Could you check a few things on this model? Use its own coordinates, in mm. Face numbers are marked on the shaded views. A direction names the side the tool comes from. Give positions to 0.01 mm unless a question says otherwise; leave off trailing zeros. Loops run counter-clockwise (first coordinate to the right, second up) from the corner with the lowest first, then second, coordinate; pieces in that order, holes last. Notation, with made-up numbers: M 17.5,-2.5 L 66.5,-2.5 A25 ccw 66.5,12.5 Z; hole C 27.25,24.5 d5. An arc over 180 degrees is marked long. Use CSV: the item, a comma, the result in double quotes.
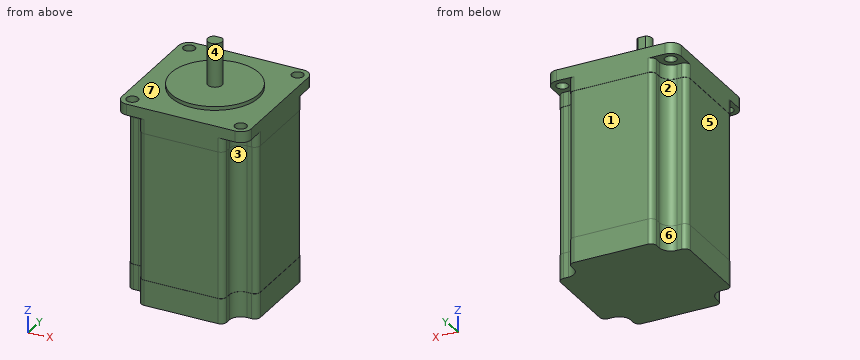
```python
from build123d import *

# Parameters (mm, degrees)
SKETCH1_R           = 3.175
BOSS_EXTRUDE1_DEPTH = 20.6
SKETCH2_R           = 19.05
BOSS_EXTRUDE2_DEPTH = 1.6
BOSS_EXTRUDE3_DEPTH = 4.8
BOSS_EXTRUDE4_DEPTH = 81.2
SKETCH7_W           = 3.420526276
SKETCH7_H           = 1.112659396
CUT_EXTRUDE5_DEPTH  = 15
CUT_EXTRUDE6_REACH  = 88
SKETCH8_R           = 2.55
CUT_EXTRUDE7_DEPTH  = 32


with BuildPart() as part:
    # Sketch1 → Boss-Extrude1 (new body)
    with BuildSketch(Plane.XY):
        Circle(SKETCH1_R)
    extrude(amount=BOSS_EXTRUDE1_DEPTH)

    # Sketch2 → Boss-Extrude2 (add)
    with BuildSketch(Plane(origin=(0, 0, 0), x_dir=(-1, 0, 0), z_dir=(0, 0, -1))):
        Circle(SKETCH2_R)
    extrude(amount=-BOSS_EXTRUDE2_DEPTH)

    # Sketch3 → Boss-Extrude3 (add)
    with BuildSketch(Plane(origin=(0, 0, 0), x_dir=(-1, 0, 0), z_dir=(0, 0, -1))):
        with BuildLine():
            Line((23.6, -28.2), (-23.6, -28.2))
            ThreePointArc((-23.6, -28.2), (-26.852691193, -26.852691193), (-28.2, -23.6))
            Line((-28.2, -23.6), (-28.2, 23.6))
            ThreePointArc((-28.2, 23.6), (-26.852691193, 26.852691193), (-23.6, 28.2))
            Line((-23.6, 28.2), (23.6, 28.2))
            ThreePointArc((23.6, 28.2), (26.852691193, 26.852691193), (28.2, 23.6))
            Line((28.2, 23.6), (28.2, -23.6))
            ThreePointArc((28.2, -23.6), (26.852691193, -26.852691193), (23.6, -28.2))
        make_face()
    extrude(amount=BOSS_EXTRUDE3_DEPTH)

    # Sketch4 → Boss-Extrude4 (add)
    with BuildSketch(Plane(origin=(0, 0, -4.8), x_dir=(-1, 0, 0), z_dir=(0, 0, -1))):
        with BuildLine():
            Line((-18.57, 23.57), (-18.57, 25.7))
            ThreePointArc((-18.57, 25.7), (-17.837766953, 27.467766953), (-16.07, 28.2))
            Line((-16.07, 28.2), (16.07, 28.2))
            ThreePointArc((16.07, 28.2), (17.837766953, 27.467766953), (18.57, 25.7))
            Line((18.57, 25.7), (18.57, 23.57))
            ThreePointArc((18.57, 23.57), (20.034466094, 20.034466094), (23.57, 18.57))
            Line((23.57, 18.57), (25.7, 18.57))
            ThreePointArc((25.7, 18.57), (27.467766953, 17.837766953), (28.2, 16.07))
            Line((28.2, 16.07), (28.2, -16.07))
            ThreePointArc((28.2, -16.07), (27.467766953, -17.837766953), (25.7, -18.57))
            Line((25.7, -18.57), (23.57, -18.57))
            ThreePointArc((23.57, -18.57), (20.034466094, -20.034466094), (18.57, -23.57))
            Line((18.57, -23.57), (18.57, -25.7))
            ThreePointArc((18.57, -25.7), (17.837766953, -27.467766953), (16.07, -28.2))
            Line((16.07, -28.2), (-16.07, -28.2))
            ThreePointArc((-16.07, -28.2), (-17.837766953, -27.467766953), (-18.57, -25.7))
            Line((-18.57, -25.7), (-18.57, -23.57))
            ThreePointArc((-18.57, -23.57), (-20.034466094, -20.034466094), (-23.57, -18.57))
            Line((-23.57, -18.57), (-25.7, -18.57))
            ThreePointArc((-25.7, -18.57), (-27.467766953, -17.837766953), (-28.2, -16.07))
            Line((-28.2, -16.07), (-28.2, 16.07))
            ThreePointArc((-28.2, 16.07), (-27.467766953, 17.837766953), (-25.7, 18.57))
            Line((-25.7, 18.57), (-23.57, 18.57))
            ThreePointArc((-23.57, 18.57), (-20.034466094, 20.034466094), (-18.57, 23.57))
        make_face()
    extrude(amount=BOSS_EXTRUDE4_DEPTH)

    # Sketch7 → Cut-Extrude5 (cut)
    with BuildSketch(Plane.XY.offset(20.6)):
        with Locations((0, 3.231329698)):
            Rectangle(SKETCH7_W, SKETCH7_H)
    extrude(amount=-CUT_EXTRUDE5_DEPTH, mode=Mode.SUBTRACT)

    # Sketch8 → Cut-Extrude6 (cut, up to next)
    with BuildSketch(Plane.XY, mode=Mode.PRIVATE) as cut_extrude6_sk1:
        with Locations((-23.57, 23.57)):
            Circle(SKETCH8_R)
    cut_extrude6_tool1 = extrude(cut_extrude6_sk1.sketch, amount=-CUT_EXTRUDE6_REACH, mode=Mode.PRIVATE) & part.part
    add(cut_extrude6_tool1.solids().sort_by_distance((-23.57, 23.57, 0))[0], mode=Mode.SUBTRACT)
    # Sketch8 → Cut-Extrude6 (cut, up to next)
    with BuildSketch(Plane.XY, mode=Mode.PRIVATE) as cut_extrude6_sk2:
        with Locations((23.57, 23.57)):
            Circle(SKETCH8_R)
    cut_extrude6_tool2 = extrude(cut_extrude6_sk2.sketch, amount=-CUT_EXTRUDE6_REACH, mode=Mode.PRIVATE) & part.part
    add(cut_extrude6_tool2.solids().sort_by_distance((23.57, 23.57, 0))[0], mode=Mode.SUBTRACT)
    # Sketch8 → Cut-Extrude6 (cut, up to next)
    with BuildSketch(Plane.XY, mode=Mode.PRIVATE) as cut_extrude6_sk3:
        with Locations((23.57, -23.57)):
            Circle(SKETCH8_R)
    cut_extrude6_tool3 = extrude(cut_extrude6_sk3.sketch, amount=-CUT_EXTRUDE6_REACH, mode=Mode.PRIVATE) & part.part
    add(cut_extrude6_tool3.solids().sort_by_distance((23.57, -23.57, 0))[0], mode=Mode.SUBTRACT)
    # Sketch8 → Cut-Extrude6 (cut, up to next)
    with BuildSketch(Plane.XY, mode=Mode.PRIVATE) as cut_extrude6_sk4:
        with Locations((-23.57, -23.57)):
            Circle(SKETCH8_R)
    cut_extrude6_tool4 = extrude(cut_extrude6_sk4.sketch, amount=-CUT_EXTRUDE6_REACH, mode=Mode.PRIVATE) & part.part
    add(cut_extrude6_tool4.solids().sort_by_distance((-23.57, -23.57, 0))[0], mode=Mode.SUBTRACT)

    # Sketch9 → Cut-Extrude7 (cut, symmetric)
    with BuildSketch(Plane.XY.offset(-43)):
        with BuildLine():
            Line((18.57, 23.57), (18.57, 25.7))
            ThreePointArc((18.57, 25.7), (17.837766953, 27.467766953), (16.07, 28.2))
            Line((16.07, 28.2), (-16.07, 28.2))
            ThreePointArc((-16.07, 28.2), (-17.837766953, 27.467766953), (-18.57, 25.7))
            Line((-18.57, 25.7), (-18.57, 23.57))
            ThreePointArc((-18.57, 23.57), (-20.034466094, 20.034466094), (-23.57, 18.57))
            Line((-23.57, 18.57), (-25.7, 18.57))
            ThreePointArc((-25.7, 18.57), (-27.467766953, 17.837766953), (-28.2, 16.07))
            Line((-28.2, 16.07), (-28.2, -16.07))
            ThreePointArc((-28.2, -16.07), (-27.467766953, -17.837766953), (-25.7, -18.57))
            Line((-25.7, -18.57), (-23.57, -18.57))
            ThreePointArc((-23.57, -18.57), (-20.034466094, -20.034466094), (-18.57, -23.57))
            Line((-18.57, -23.57), (-18.57, -25.7))
            ThreePointArc((-18.57, -25.7), (-17.837766953, -27.467766953), (-16.07, -28.2))
            Line((-16.07, -28.2), (16.07, -28.2))
            ThreePointArc((16.07, -28.2), (17.837766953, -27.467766953), (18.57, -25.7))
            Line((18.57, -25.7), (18.57, -23.57))
            ThreePointArc((18.57, -23.57), (20.034466094, -20.034466094), (23.57, -18.57))
            Line((23.57, -18.57), (25.7, -18.57))
            ThreePointArc((25.7, -18.57), (27.467766953, -17.837766953), (28.2, -16.07))
            Line((28.2, -16.07), (28.2, 16.07))
            ThreePointArc((28.2, 16.07), (27.467766953, 17.837766953), (25.7, 18.57))
            Line((25.7, 18.57), (23.57, 18.57))
            ThreePointArc((23.57, 18.57), (20.034466094, 20.034466094), (18.57, 23.57))
        make_face()
        with BuildLine():
            Line((18.47, 23.57), (18.47, 25.7))
            ThreePointArc((18.47, 25.7), (17.767056275, 27.397056275), (16.07, 28.1))
            Line((16.07, 28.1), (-16.07, 28.1))
            ThreePointArc((-16.07, 28.1), (-17.767056275, 27.397056275), (-18.47, 25.7))
            Line((-18.47, 25.7), (-18.47, 23.57))
            ThreePointArc((-18.47, 23.57), (-19.963755416, 19.963755416), (-23.57, 18.47))
            Line((-23.57, 18.47), (-25.7, 18.47))
            ThreePointArc((-25.7, 18.47), (-27.397056275, 17.767056275), (-28.1, 16.07))
            Line((-28.1, 16.07), (-28.1, -16.07))
            ThreePointArc((-28.1, -16.07), (-27.397056275, -17.767056275), (-25.7, -18.47))
            Line((-25.7, -18.47), (-23.57, -18.47))
            ThreePointArc((-23.57, -18.47), (-19.963755416, -19.963755416), (-18.47, -23.57))
            Line((-18.47, -23.57), (-18.47, -25.7))
            ThreePointArc((-18.47, -25.7), (-17.767056275, -27.397056275), (-16.07, -28.1))
            Line((-16.07, -28.1), (16.07, -28.1))
            ThreePointArc((16.07, -28.1), (17.767056275, -27.397056275), (18.47, -25.7))
            Line((18.47, -25.7), (18.47, -23.57))
            ThreePointArc((18.47, -23.57), (19.963755416, -19.963755416), (23.57, -18.47))
            Line((23.57, -18.47), (25.7, -18.47))
            ThreePointArc((25.7, -18.47), (27.397056275, -17.767056275), (28.1, -16.07))
            Line((28.1, -16.07), (28.1, 16.07))
            ThreePointArc((28.1, 16.07), (27.397056275, 17.767056275), (25.7, 18.47))
            Line((25.7, 18.47), (23.57, 18.47))
            ThreePointArc((23.57, 18.47), (19.963755416, 19.963755416), (18.47, 23.57))
        make_face(mode=Mode.SUBTRACT)
    extrude(amount=CUT_EXTRUDE7_DEPTH, both=True, mode=Mode.SUBTRACT)


solid = part.part
```
1. I want a section at B-B, the plane x = 0. List the corners of the cut face in (y, z) for me (3 decimals).
Outcome:
outline,"M -28.2,-86 L 28.2,-86 L 28.2,-75 L 28.1,-75 L 28.1,-11 L 28.2,-11 L 28.2,0 L 19.05,0 L 19.05,1.6 L 3.175,1.6 L 3.175,5.6 L 2.675,5.6 L 2.675,20.6 L -3.175,20.6 L -3.175,1.6 L -19.05,1.6 L -19.05,0 L -28.2,0 L -28.2,-11 L -28.1,-11 L -28.1,-75 L -28.2,-75 Z"
2. I'm going to push flat-ended pins straight in: pin 1 Ø8 at (y, z) = (4.5, -38.5) entering from -X; pin 2 Ø1.7 at (x, z) = (-25, -83) entering from +Y; pin 3 Ø1.7 at (x, z) = (-24.5, -40.5) entering from -Y; pin 4 Ø4 at (x, y) = (-23.57, -23.57) entering from +Z. Where does each tip first touch, or does it pass through?
Outcome:
pin 1,"x = -28.1"
pin 2,"y = 18.57"
pin 3,"y = -18.47"
pin 4,"through"
3. I want a section at A-A, the plane z = -17. List the corners of the cut face in (x, y) for me.
Outcome:
outline,"M -28.1,-16.07 A2.4 ccw -25.7,-18.47 L -23.57,-18.47 A5.1 cw -18.47,-23.57 L -18.47,-25.7 A2.4 ccw -16.07,-28.1 L 16.07,-28.1 A2.4 ccw 18.47,-25.7 L 18.47,-23.57 A5.1 cw 23.57,-18.47 L 25.7,-18.47 A2.4 ccw 28.1,-16.07 L 28.1,16.07 A2.4 ccw 25.7,18.47 L 23.57,18.47 A5.1 cw 18.47,23.57 L 18.47,25.7 A2.4 ccw 16.07,28.1 L -16.07,28.1 A2.4 ccw -18.47,25.7 L -18.47,23.57 A5.1 cw -23.57,18.47 L -25.7,18.47 A2.4 ccw -28.1,16.07 Z"
4. Please list where these lines run through material, in increasing order: line 1 (Y direction, x = -23.57, z = -1.4); line 2 (Y direction, x = -23, z = -3); line 3 (X direction, y = -3, z = -27).
Outcome:
line 1,"-28.2 to -26.12, -21.02 to 21.02, 26.12 to 28.2"
line 2,"-28.2 to -26.06, -21.08 to 21.08, 26.06 to 28.2"
line 3,"-28.1 to 28.1"
5. I want a section at D-D, the plane x = 13. List the corners of the cut face in (y, z) for me, then the cut area to 3 significant figures.
Outcome:
outline,"M -28.2,-86 L 28.2,-86 L 28.2,-75 L 28.1,-75 L 28.1,-11 L 28.2,-11 L 28.2,0 L 13.92,0 L 13.92,1.6 L -13.92,1.6 L -13.92,0 L -28.2,0 L -28.2,-11 L -28.1,-11 L -28.1,-75 L -28.2,-75 Z"
area,"4,880 mm2"
6. I want a section at C-C, the plane y = 0. List the corners of the cut face in (x, z) for me (3 decimals), then the cut area to 3 significant figures.
Outcome:
outline,"M -28.2,-86 L 28.2,-86 L 28.2,-75 L 28.1,-75 L 28.1,-11 L 28.2,-11 L 28.2,0 L 19.05,0 L 19.05,1.6 L 3.175,1.6 L 3.175,20.6 L -3.175,20.6 L -3.175,1.6 L -19.05,1.6 L -19.05,0 L -28.2,0 L -28.2,-11 L -28.1,-11 L -28.1,-75 L -28.2,-75 Z"
area,"5,020 mm2"
7. If we mould it in two halves opening along Z, with no side actions, what happens to the marked faces 5, 6 and 7? For each: +Z half, -Z half, draft (parallel to the pull), parting line (faces both ways), or undercut.
Outcome:
face 5,"undercut"
face 6,"draft"
face 7,"+Z half"
8. Which directions (+Z, -Z, +X, -X, +Y, -Y) give clear straight access to the entire face, cutting with the end or side of a thin tool? Please do the marked faces 1, 2, 3 and 4.
Outcome:
face 1,"+X, -X, +Y"
face 2,"-X, +Y"
face 3,"+X, -Y"
face 4,"+Z"
